```python
from build123d import *

# Parameters (mm, degrees)
BOSS_EXTRUDE1_DEPTH = 5
FILLET1_R           = 1
BOSS_EXTRUDE2_DEPTH = 13
CUT_EXTRUDE1_DEPTH  = 143.017604543


with BuildPart() as part:
    # Sketch1 → Boss-Extrude1 (new body)
    with BuildSketch(Plane(origin=(0, 0, 0), x_dir=(1, 0, 0), z_dir=(0, 1, 0))):
        with BuildLine():
            Line((5, 0), (95, 0))
            ThreePointArc((95, 0), (98.535533906, 1.464466094), (100, 5))
            Line((100, 5), (100, 95))
            ThreePointArc((100, 95), (98.535533906, 98.535533906), (95, 100))
            Line((95, 100), (5, 100))
            ThreePointArc((5, 100), (1.464466094, 98.535533906), (0, 95))
            Line((0, 95), (0, 5))
            ThreePointArc((0, 5), (1.464466094, 1.464466094), (5, 0))
        make_face()
    extrude(amount=BOSS_EXTRUDE1_DEPTH)

    # Fillet1
    fillet1_edges = [part.edges().sort_by_distance(p)[0] for p in [
        (1.464466094, 5, -98.535533906),
        (0, 5, -50),
        (1.464466094, 5, -1.464466094),
        (50, 5, 0),
        (98.535533906, 5, -1.464466094),
        (100, 5, -50),
        (98.535533906, 5, -98.535533906),
        (50, 5, -100),
    ]]
    fillet(fillet1_edges, radius=FILLET1_R)

    # Sketch2 → Boss-Extrude2 (add)
    with BuildSketch(Plane(origin=(0, 5, 0), x_dir=(1, 0, 0), z_dir=(0, 1, 0))):
        Polygon((70, 50), (64.142135624, 64.142135624), (50, 70), (35.857864376, 64.142135624), (30, 50), (35.857864376, 35.857864376), (50, 30), (64.142135624, 35.857864376), align=None)
        Polygon((68, 50), (62.727922061, 62.727922061), (50, 68), (37.272077939, 62.727922061), (32, 50), (37.272077939, 37.272077939), (50, 32), (62.727922061, 37.272077939), align=None, mode=Mode.SUBTRACT)
    extrude(amount=BOSS_EXTRUDE2_DEPTH)

    # Sketch5 → Cut-Extrude1 (cut, through all)
    with BuildSketch(Plane(origin=(0, 5, 0), x_dir=(1, 0, 0), z_dir=(0, 1, 0))):
        Polygon((68, 50), (62.727922061, 62.727922061), (50, 68), (37.272077939, 62.727922061), (32, 50), (37.272077939, 37.272077939), (50, 32), (62.727922061, 37.272077939), align=None)
    extrude(amount=-CUT_EXTRUDE1_DEPTH, mode=Mode.SUBTRACT)


solid = part.part
```
Verification items for the finished model (mm, model axes). A direction names the side the tool comes from. Give positions to 0.01 mm unless a question says otherwise; leave off trailing zeros. Order: outer loops, then holes, each group sorted by start corner. A loop starts at its lowest first (then second) coordinate and runs counter-clockwise, first axis right, second up. Notation, with made-up numbers: M 20,37.25 L 67,37.25 A24 ccw 67,66.25 Z; hole C 66,-26.5 d9. An arc over 180 degrees is marked long. Return JSON: item names as keys, results as strings. Group by question number.
1) Go/stop test with flat-tipped pins: pin 1 Ø6 at (x, y) = (38, 9) entering from +Z; pin 2 Ø1.5 at (y, z) = (12, -57) entering from +X. Record where each tip stops, or that it passes through.
2) Scan lines: line 1 (Y direction, x = 23, z = -25); line 2 (Z direction, x = 64, y = 9.5); line 3 (Z direction, x = 52.5, y = 2.5). Record each from-to range of solid material in increasing order.
3) Section check A-A on y = 11.75. Record the cut outline in (x, z).
4) Access from +Z, -Z, +X, -X, +Y, -Y to the whole of each face (thin tool, end or side, straight path). Record for faces 4 (the face through (56.45, 9.13, -65.33)), 5 (the face through (43, 11.4, -67.1)), 6 (the face through (57, 11.4, -32.9)).
5) Mould release check, pull along X, two halves, no side actions. Record for faces 1 (the face through (32.9, 11.4, -43)), 2 (the face through (49, 2, 0)), 3 (the face through (56.275, 9.126, -34.599)): pulls with the +X half, pulls with the -X half, needs draft (parallel to the pull), parting line crosses it, or undercut.
6) Section check D-D on z = -25. Record the cut outline in (x, y).
7) Section check C-C on x = 53.5. Record the cut outline in (y, z).
8) Section check B-B on z = -54. Record the cut outline in (x, y).
Answer block:
{
 "1": {"pin 1": "stops at z = -33.73", "pin 2": "stops at x = 67.41"},
 "2": {"line 1": "y = 0 to 5", "line 2": "z = -64.2 to -59.66, -40.34 to -35.8", "line 3": "z = -100 to -66.96, -33.04 to 0"},
 "3": {"outline": "M 30,-50 L 35.86,-64.14 L 50,-70 L 64.14,-64.14 L 70,-50 L 64.14,-35.86 L 50,-30 L 35.86,-35.86 Z; hole M 32,-50 L 37.27,-62.73 L 50,-68 L 62.73,-62.73 L 68,-50 L 62.73,-37.27 L 50,-32 L 37.27,-37.27 Z"},
 "4": {"face 4": "+Y, -Y", "face 5": "-Z, -X, +Y", "face 6": "+Z, +X, +Y"},
 "5": {"face 1": "pulls with the -X half", "face 2": "needs draft", "face 3": "undercut"},
 "6": {"outline": "M 0,0 L 100,0 L 100,4 A1 ccw 99,5 L 1,5 A1 ccw 0,4 Z"},
 "7": {"outline": "M 0,-100 L 4,-100 A1 ccw 5,-99 L 5,-68.55 L 18,-68.55 L 18,-66.55 L 0,-66.55 Z; M 0,-33.45 L 18,-33.45 L 18,-31.45 L 5,-31.45 L 5,-1 A1 ccw 4,0 L 0,0 Z"},
 "8": {"outline": "M 0,0 L 33.66,0 L 33.66,18 L 31.66,18 L 31.66,5 L 1,5 A1 ccw 0,4 Z; M 66.34,0 L 100,0 L 100,4 A1 ccw 99,5 L 68.34,5 L 68.34,18 L 66.34,18 Z"}
}
